Could you check a few things on this model? Use its own coordinates, in mm. Face numbers are marked on the shaded views. A direction names the side the tool comes from. Round coordinates to 2 decimals unless told otherwise and drop trailing zeros. Write each loop counter-clockwise with the first axis right and the second up, starting at its lowest first coordinate (ties: lowest second). Pieces come first, ordered by that corner, then holes. Notation, with made-up numbers: (-22, 9.25) - (-12, 9.25) arc R11 ccw to (-12, 14.25) - close; hole circle Ø6 at (9.5, -6). An arc over 180 degrees is marked (long way). Put each result on its own line as item: value.
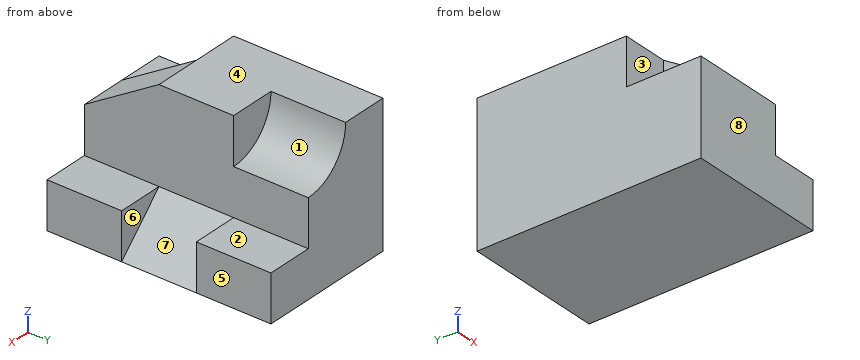
from build123d import *

# Parameters (mm, degrees)
F1_DEPTH = 24
F3_DEPTH = 8
F5_DEPTH = 30.001
F6_DEPTH = 10
F7_R     = 10
F8_DEPTH = 16


with BuildPart() as f1:
    # F0 (on Front) → F1 (new body, symmetric)
    with BuildSketch(Plane.XZ):
        Polygon((0, 30), (0, 0), (30, 0), (30, 10), (20, 10), (20, 30), align=None)
    extrude(amount=F1_DEPTH, both=True)

    # F2 (on Front) → F3 (cut, symmetric)
    with BuildSketch(Plane.XZ):
        Polygon((30, 0), (30, 10), (20, 10), align=None)
    extrude(amount=F3_DEPTH, both=True, mode=Mode.SUBTRACT)

    # F4 (on face) → F5 (cut, through all)
    with BuildSketch(Plane(origin=(0, 0, 0), x_dir=(0, -1, 0), z_dir=(-1, 0, 0))):
        Polygon((24, 20), (24, 30), (8, 30), align=None)
    extrude(amount=-F5_DEPTH, mode=Mode.SUBTRACT)

    # F4 (on face) → F6 (cut)
    with BuildSketch(Plane(origin=(0, 0, 0), x_dir=(0, -1, 0), z_dir=(-1, 0, 0))):
        Polygon((24, 20), (8, 30), (8, 20), align=None)
    extrude(amount=-F6_DEPTH, mode=Mode.SUBTRACT)

    # F7 (on face) → F8 (cut)
    with BuildSketch(Plane(origin=(0, 24, 0), x_dir=(-1, 0, 0), z_dir=(0, 1, 0))):
        with Locations((-20, 30)):
            Circle(F7_R)
    extrude(amount=-F8_DEPTH, mode=Mode.SUBTRACT)


solid = f1.part
(1) Please list where these lines run through material, in increasing order: probe 1 along Y at (x, z) = (26.75, 6.5); probe 2 along Y at (x, z) = (5.75, 22); probe 3 along Z at (x, y) = (27, 9). Write a range as from..to.
Values found:
probe 1: y = -24..-8, 8..24
probe 2: y = -8..24
probe 3: z = 0..10
(2) For the marked faces 1, 2, 3 and 4, which set-ups out of +Z, -Z, +X, -X, +Y, -Y let a thin tool reach every point of the face, with its end or its side?
Values found:
face 1: +Z, +X, +Y
face 2: +Z, +X, +Y, -Y
face 3: +Z, -X, -Y
face 4: +Z, +X, -X, +Y, -Y
(3) Imagine slicing it at C-C, the plane y = 16.5. List the corners of the cut face in (x, z) for me, then the cut area to 3 significant figures.
Values found:
outline: (0, 0) - (30, 0) - (30, 10) - (20, 10) - (20, 20) arc R10 cw to (10, 30) - (0, 30) - close
area: 621 mm^2
(4) If we mould it in two halves opening along Y, with no side actions, what happens to the marked faces 5, 6, 7 and 8? For each: pulls with the +Y half, pulls with the -Y half, needs draft (parallel to the pull), parting line crosses it, or undercut.
Values found:
face 5: needs draft
face 6: undercut
face 7: undercut
face 8: pulls with the -Y half
(5) I'm going to push flat-ended pins straight in: pin 1 (16 mm diameter, centred on y = -10.5, z = 21, fed in from +X); pin 2 (5 mm diameter, centred on x = 4, y = -14, fed in from +Z); pin 3 (8 mm diameter, centred on x = 17, z = 26.5, fed in from +Y). Where does each tip first touch, or does it pass through?
Values found:
pin 1: stops at x = 20
pin 2: stops at z = 20
pin 3: stops at y = 8
(6) Imagine slicing it at A-A, the plane z = 4.75. List the corners of the cut face in (x, y) for me, then the cut area to 3 significant figures.
Values found:
outline: (0, -24) - (30, -24) - (30, -8) - (25.25, -8) - (25.25, 8) - (30, 8) - (30, 24) - (0, 24) - close
area: 1,360 mm^2
(7) Imagine slicing it at D-D, the plane x = 2.5. List the corners of the cut face in (y, z) for me.
Values found:
outline: (-24, 0) - (24, 0) - (24, 30) - (-8, 30) - (-8, 20) - (-24, 20) - close
(8) Imagine slicing it at B-B, the plane x = 22.5. List the corners of the cut face in (y, z) for me, then the cut area to 3 significant figures.
Values found:
outline: (-24, 0) - (24, 0) - (24, 10) - (8, 10) - (8, 7.5) - (-8, 7.5) - (-8, 10) - (-24, 10) - close
area: 440 mm^2
